Source: CAD feature listing. Evaluate the final solid. Frame: model axes, mm. Coordinates: 2 decimals unless noted, no trailing zeros. Order: outer loops, then holes, each group sorted by start corner. A loop starts at its lowest first (then second) coordinate and runs counter-clockwise, first axis right, second up.
```python
from build123d import *

# Parameters (mm, degrees)
F0_R     = 12.4344228223
F1_DEPTH = 12.7
F2_SIZE  = 1
F3_T     = -1.5


# Not quite as in the source:
# - a fillet or chamfer that OpenCascade refuses, or shapes differently, is made with other operations: its cross-section is extruded or revolved along the edge and cut away or added
# - the program builds the solid bodies; features that only make, move or delete a surface that nothing else refers to are left out


with BuildPart() as f1:
    # F0 (on Front) → F1 (new body)
    with BuildSketch(Plane.XZ):
        Circle(F0_R)
    extrude(amount=F1_DEPTH)

    # F2
    f2_edges = [f1.edges().sort_by_distance(p)[0] for p in [
        (-12.434423, 0, 0),
        (12.434423, -6.35, 0),
        (-12.434423, -12.7, 0),
    ]]
    chamfer(f2_edges, length=F2_SIZE)

    # F3
    f3_openings = [f1.faces().sort_by_distance(p)[0] for p in [
        (0, 0, 0),
    ]]
    offset(amount=F3_T, openings=f3_openings)

    # F5: chamfer of 0.2 on 2 edges, made by hand

    # F5_s1 → F5_t2 (revolve, cut)
    with BuildSketch(Plane.XY):
        Polygon((9.5131024788, 0), (9.454523835, -0.1414213562), (9.3131024788, 0), align=None)
    revolve(axis=Axis((0, 0, 0), (0, 1, 0)), mode=Mode.SUBTRACT)


solid = f1.part
```
Q1. Material intervals for line 1 along Z through (x, y) = (0, -4.75); line 2 along Y through (x, z) = (4, -5.5); line 3 along Z through (x, y) = (7.75, -5.5), sorted ascending.
Solutions:
line 1: z = -12.43 to -10.93, 10.93 to 12.43
line 2: y = -12.7 to -11.2
line 3: z = -9.72 to -7.71, 7.71 to 9.72
Q2. Pull-direction query (X, two-part tool) for faces 1 (the cylindrical face through (-12.422, -6.275, 0.547)), 2 (the flat face through (-4, 0, 9)), 3 (the cylindrical face through (10.43, -6.28, 3.28)), 4 (the flat face through (0, -11.2, 0)); classes: pulls with the +X half, pulls with the -X half, needs draft (parallel to the pull), parting line crosses it, or undercut.
Solutions:
face 1: parting line crosses it
face 2: needs draft
face 3: undercut
face 4: undercut
Q3. Pin query (flat end, axial travel): P1, Ø6, axis at y = -9, z = -1, coming from the -X side; P2, Ø2, axis at x = 6, y = -3.5, coming from the -Z side; P3, Ø4, axis at x = 6.5, z = 3.5, coming from the +Y side. Return the tip coordinate at first contact, or that it passes through.
Solutions:
P1: stops at x = -12.43
P2: stops at z = -11.38
P3: stops at y = -11.2
Q4. Section query B-B on z = 0. Output: boundary loops of the cut face in (x, y), plus the area to 3 significant figures.
Solutions:
outline: (-12.43, -11.7) - (-11.43, -12.7) - (11.43, -12.7) - (12.43, -11.7) - (12.43, -1) - (11.43, 0) - (9.51, 0) - (9.45, -0.14) - (10.93, -1.62) - (10.93, -11.08) - (10.81, -11.2) - (-10.81, -11.2) - (-10.93, -11.08) - (-10.93, -1.62) - (-9.45, -0.14) - (-9.51, 0) - (-11.43, 0) - (-12.43, -1) - close
area: 71.5 mm2
Q5. Section query C-C on x = 0. Output: boundary loops of the cut face in (y, z).
Solutions:
outline: (-12.7, -11.43) - (-11.7, -12.43) - (-1, -12.43) - (0, -11.43) - (0, -9.51) - (-0.14, -9.45) - (-1.62, -10.93) - (-11.08, -10.93) - (-11.2, -10.81) - (-11.2, 10.81) - (-11.08, 10.93) - (-1.62, 10.93) - (-0.14, 9.45) - (0, 9.51) - (0, 11.43) - (-1, 12.43) - (-11.7, 12.43) - (-12.7, 11.43) - close
Q6. Section query A-A on y = -4.75. Output: boundary loops of the cut face in (x, z).
Solutions:
outline: circle Ø24.87 at (0, 0); hole circle Ø21.87 at (0, 0)
